from build123d import *

# Parameters (mm, degrees)
SKETCH1_W           = 16
SKETCH1_H           = 25.5
SKETCH1_R           = 1.1
BASE_FLANGE1_DEPTH  = 1.57
EDGE_FLANGE2_DEPTH  = 25.5
EDGE_FLANGE3_DEPTH  = 25.5
SKETCH23_W          = 1.57
SKETCH23_H          = 9.77
BOSS_EXTRUDE1_DEPTH = 9
CUT_EXTRUDE1_DEPTH  = 33.18625483
SKETCH29_R          = 1.1
CUT_EXTRUDE2_DEPTH  = 33.18625483


# Sheet-metal steps are written as plain solids
with BuildPart() as part:
    # Sketch1 → Base-Flange1 (new body)
    with BuildSketch(Plane(origin=(0, 0, 0), x_dir=(1, 0, 0), z_dir=(0, 1, 0))):
        Rectangle(SKETCH1_W, SKETCH1_H)
        with Locations(Location((-5, 9.75, 0), (0, 0, 270))):
            Circle(SKETCH1_R, mode=Mode.SUBTRACT)
        with Locations(Location((5, 9.75, 0), (0, 0, 270))):
            Circle(SKETCH1_R, mode=Mode.SUBTRACT)
        with Locations(Location((-5, -9.75, 0), (0, 0, 270))):
            Circle(SKETCH1_R, mode=Mode.SUBTRACT)
        with Locations(Location((5, -9.75, 0), (0, 0, 270))):
            Circle(SKETCH1_R, mode=Mode.SUBTRACT)
    extrude(amount=-BASE_FLANGE1_DEPTH)

    # Edge-Flange2 section (across the edge) → Edge-Flange2 (add)
    with BuildSketch(Plane(origin=(9, 0, 12.75), x_dir=(-1, 0, 0), z_dir=(0, 0, -1))):
        with BuildLine():
            Line((-1.57, 1), (-1.57, 10.77))
            Line((-1.57, 10.77), (0, 10.77))
            Line((0, 10.77), (0, 1))
            ThreePointArc((0, 1), (0.292893219, 0.292893219), (1, 0))
            Line((1, 0), (1, -1.57))
            ThreePointArc((1, -1.57), (-0.817264428, -0.817264428), (-1.57, 1))
        make_face()
    extrude(amount=EDGE_FLANGE2_DEPTH)

    # Edge-Flange3 section (across the edge) → Edge-Flange3 (add)
    with BuildSketch(Plane(origin=(-9, 0, -12.75), x_dir=(1, 0, 0), z_dir=(0, 0, 1))):
        with BuildLine():
            Line((-1.57, 1), (-1.57, 10.77))
            Line((-1.57, 10.77), (0, 10.77))
            Line((0, 10.77), (0, 1))
            ThreePointArc((0, 1), (0.292893219, 0.292893219), (1, 0))
            Line((1, 0), (1, -1.57))
            ThreePointArc((1, -1.57), (-0.817264428, -0.817264428), (-1.57, 1))
        make_face()
    extrude(amount=EDGE_FLANGE3_DEPTH)

    # Sketch23 → Boss-Extrude1 (add)
    with BuildSketch(Plane.XY.offset(12.75)):
        with Locations((-9.785, 5.885)):
            Rectangle(SKETCH23_W, SKETCH23_H)
        with Locations((9.785, 5.885)):
            Rectangle(SKETCH23_W, SKETCH23_H)
    extrude(amount=BOSS_EXTRUDE1_DEPTH)

    # Sketch24 → Cut-Extrude1 (cut, through all)
    with BuildSketch(Plane(origin=(10.57, 0, 0), x_dir=(0, 0, -1), z_dir=(1, 0, 0))):
        Polygon((-21.75, 10.77), (-21.75, 1), (-15.25, 1), (-20.25, 4.27), align=None)
    extrude(amount=-CUT_EXTRUDE1_DEPTH, mode=Mode.SUBTRACT)

    # Sketch29 → Cut-Extrude2 (cut, through all)
    with BuildSketch(Plane(origin=(10.57, 0, 0), x_dir=(0, 0, -1), z_dir=(1, 0, 0))):
        with Locations(Location((-19.288461538, 8.77, 0), (0, 0, 90))):
            Circle(SKETCH29_R)
        with Locations(Location((10.711538462, 8.77, 0), (0, 0, 90))):
            Circle(SKETCH29_R)
    extrude(amount=-CUT_EXTRUDE2_DEPTH, mode=Mode.SUBTRACT)


solid = part.part
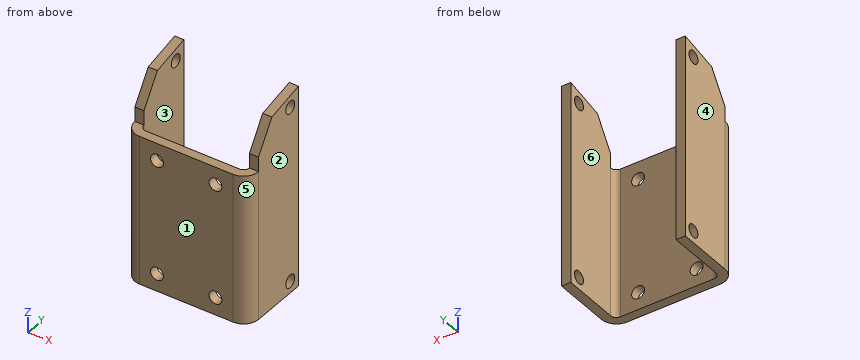
Work out the finished part from the listing and answer in its coordinate system (mm). Face numbers are marked on the shaded views. A direction names the side the tool comes from. Give positions to 0.01 mm unless a question says otherwise; leave off trailing zeros. Loops run counter-clockwise (first coordinate to the right, second up) from the corner with the lowest first, then second, coordinate; pieces in that order, holes last. Notation, with made-up numbers: (23, 65.5) -> (60, 65.5) arc R18 ccw to (60, 73.5) -> close; hole circle Ø11 at (-5.75, -10). An arc over 180 degrees is marked (long way). Use a Markdown table: item, result. Add a question column.
1) For a pull along X with two mould halves and no side action, classify the marked faces 1, 2, 3 and 4 as +X half, -X half, draft (parallel to the pull), parting line (faces both ways), or undercut.
2) Each of these flat-tipped pins is pushed along its axis until it touches: P1, Ø0.5, axis at x = -10, z = 14.5, coming from the -Y side; P2, Ø3, axis at x = -5, z = 9.75, coming from the +Y side; P3, Ø2, axis at x = 5, z = -9.75, coming from the -Y side; P4, Ø6, axis at x = -5, y = 2.5, coming from the +Z side. Where does it stop, or does it pass through?
3) The part is cut by section D-D, the plane z = 17.5. Determine the outline of the cut face in (x, y).
4) The part is cut by section A-A, the plane z = 9.75. Determine the outline of the cut face in (x, y).
5) Which of the six approach directions +Z, -Z, +X, -X, +Y, -Y give full straight-line access (tool end or side, diameter ignored) to the marked faces 5 and 6?
6) Consider line 1 along X through (y, z) = (4, 8.5); line 2 along X through (y, z) = (-0.9, -9.75); line 3 along X through (y, z) = (-0.75, -9.75). Determine where each line is inside the solid, lowest interval first.
7) The part is cut by section C-C, the plane y = 9.5. Determine the outline of the cut face in (x, z).
8) The part is cut by section B-B, the plane x = 5. Determine the outline of the cut face in (y, z).
Reported:
| question | item | result |
|---|---|---|
| 1 | face 1 | draft |
| 1 | face 2 | +X half |
| 1 | face 3 | undercut |
| 1 | face 4 | -X half |
| 2 | P1 | stops at y = 1 |
| 2 | P2 | stops at y = 0 |
| 2 | P3 | passes through |
| 2 | P4 | stops at z = 12.75 |
| 3 | outline | (-10.57, 2.47) -> (-9, 2.47) -> (-9, 10.77) -> (-10.57, 10.77) -> close; (9, 2.47) -> (10.57, 2.47) -> (10.57, 10.77) -> (9, 10.77) -> close |
| 4 | outline | (-10.57, 1) arc R2.57 ccw to (-8, -1.57) -> (-6.1, -1.57) -> (-6.1, 0) -> (-8, 0) arc R1 cw to (-9, 1) -> (-9, 10.77) -> (-10.57, 10.77) -> close; (-3.9, -1.57) -> (3.9, -1.57) -> (3.9, 0) -> (-3.9, 0) -> close; (6.1, -1.57) -> (8, -1.57) arc R2.57 ccw to (10.57, 1) -> (10.57, 10.77) -> (9, 10.77) -> (9, 1) arc R1 cw to (8, 0) -> (6.1, 0) -> close |
| 5 | face 5 | +Z, -Z, +X, -Y |
| 5 | face 6 | +Z, -Z, +Y |
| 6 | line 1 | x = -10.57 to -9, 9 to 10.57 |
| 6 | line 2 | x = -9.73 to -6.1, -3.9 to 3.9, 6.1 to 9.73 |
| 6 | line 3 | x = -9.88 to -6.1, -3.9 to 3.9, 6.1 to 9.88 |
| 7 | outline | (-10.57, -12.75) -> (-9, -12.75) -> (-9, -11.53) -> (-10.57, -11.53) -> close; (-10.57, -9.89) -> (-9, -9.89) -> (-9, 18.47) -> (-10.57, 18.47) -> close; (-10.57, 20.11) -> (-9, 20.11) -> (-9, 21.46) -> (-10.57, 21.46) -> close; (9, -12.75) -> (10.57, -12.75) -> (10.57, -11.53) -> (9, -11.53) -> close; (9, -9.89) -> (10.57, -9.89) -> (10.57, 18.47) -> (9, 18.47) -> close; (9, 20.11) -> (10.57, 20.11) -> (10.57, 21.46) -> (9, 21.46) -> close |
| 8 | outline | (-1.57, -12.75) -> (0, -12.75) -> (0, -10.85) -> (-1.57, -10.85) -> close; (-1.57, -8.65) -> (0, -8.65) -> (0, 8.65) -> (-1.57, 8.65) -> close; (-1.57, 10.85) -> (0, 10.85) -> (0, 12.75) -> (-1.57, 12.75) -> close |
